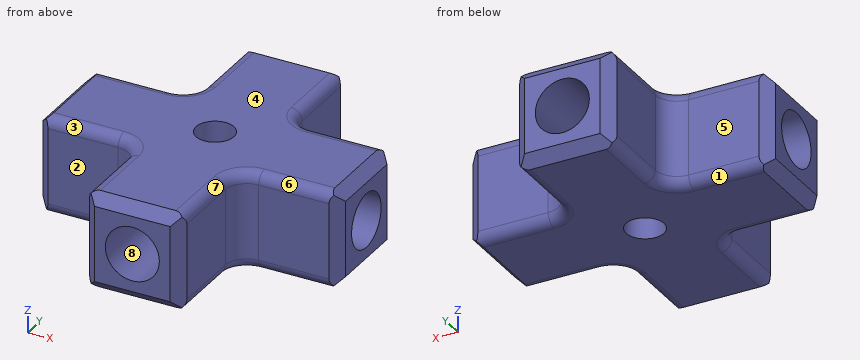
```python
from build123d import *

# Parameters (mm, degrees)
F0_W     = 9
F0_H     = 9.5
F0_W_2   = 9.5
F0_H_2   = 9
F0_R     = 1.75
F1_DEPTH = 9
F4_R     = 2.5
F6_DEPTH = 6.5
F3_R     = 2.5
F7_DEPTH = 6.5
F5_R     = 2.5
F8_DEPTH = 6.5
F2_R     = 2.5
F9_DEPTH = 6.5
F10_R    = 2
F11_SIZE = 1
F12_R    = 1


with BuildPart() as f1:
    # F0 (on Top) → F1 (new body)
    with BuildSketch(Plane.XY):
        with Locations((0, -9.25)):
            Rectangle(F0_W, F0_H)
        with Locations((9.25, 0)):
            Rectangle(F0_W_2, F0_H_2)
        with Locations((-9.25, 0)):
            Rectangle(F0_W_2, F0_H_2)
        with Locations((0, 9.25)):
            Rectangle(F0_W, F0_H)
        Rectangle(F0_W, F0_H_2)
        Circle(F0_R, mode=Mode.SUBTRACT)
    extrude(amount=F1_DEPTH)

    # F4 (on face) → F6 (cut)
    with BuildSketch(Plane(origin=(-14, 0, 0), x_dir=(0, -1, 0), z_dir=(-1, 0, 0))):
        with Locations((0, 4.4999998063)):
            Circle(F4_R)
    extrude(amount=-F6_DEPTH, mode=Mode.SUBTRACT)

    # F3 (on face) → F7 (cut)
    with BuildSketch(Plane.YZ.offset(14)):
        with Locations((0, 4.5)):
            Circle(F3_R)
    extrude(amount=-F7_DEPTH, mode=Mode.SUBTRACT)

    # F5 (on face) → F8 (cut)
    with BuildSketch(Plane.XZ.offset(14)):
        with Locations((0, 4.5042946003)):
            Circle(F5_R)
    extrude(amount=-F8_DEPTH, mode=Mode.SUBTRACT)

    # F2 (on face) → F9 (cut)
    with BuildSketch(Plane(origin=(0, 14, 0), x_dir=(-1, 0, 0), z_dir=(0, 1, 0))):
        with Locations((0, 4.5)):
            Circle(F2_R)
    extrude(amount=-F9_DEPTH, mode=Mode.SUBTRACT)

    # F10
    f10_edges = [f1.edges().sort_by_distance(p)[0] for p in [
        (-4.5, 4.5, 4.5),
        (-4.5, -4.5, 4.5),
        (4.5, -4.5, 4.5),
        (4.5, 4.5, 4.5),
    ]]
    fillet(f10_edges, radius=F10_R)

    # F11
    f11_edges = [f1.edges().sort_by_distance(p)[0] for p in [
        (14, 4.5, 4.5),
        (4.5, 14, 4.5),
        (-4.5, 14, 4.5),
        (-14, 4.5, 4.5),
        (-14, -4.5, 4.5),
        (-4.5, -14, 4.5),
        (4.5, -14, 4.5),
        (14, -4.5, 4.5),
        (14, 0, 0),
        (0, 14, 0),
        (-14, 0, 0),
        (0, -14, 0),
        (-14, 0, 9),
        (0, 14, 9),
        (0, -14, 9),
        (14, 0, 9),
    ]]
    chamfer(f11_edges, length=F11_SIZE)

    # F12
    f12_edges = [f1.edges().sort_by_distance(p)[0] for p in [
        (-9.75, -4.5, 9),
        (-9.75, 4.5, 9),
        (-4.5, -9.75, 9),
        (4.5, -9.75, 9),
        (9.75, -4.5, 9),
        (9.75, 4.5, 9),
        (4.5, 9.75, 9),
        (-4.5, 9.75, 9),
        (-9.75, 4.5, 0),
        (-9.75, -4.5, 0),
        (-4.5, -9.75, 0),
        (4.5, -9.75, 0),
        (9.75, -4.5, 0),
        (9.75, 4.5, 0),
        (4.5, 9.75, 0),
        (-4.5, 9.75, 0),
    ]]
    fillet(f12_edges, radius=F12_R)


solid = f1.part
```
Geometry: final body of the model. Coordinates: model frame, mm. Face numbers are marked on the shaded views. A direction names the side the tool comes from. Coordinates: 2 decimals unless noted, no trailing zeros. Order: outer loops, then holes, each group sorted by start corner. A loop starts at its lowest first (then second) coordinate and runs counter-clockwise, first axis right, second up. Notation, with made-up numbers: (37, 8) -> (58, 8) arc R25 cw to (58, 21) -> close; hole circle Ø10 at (7, 72.25). An arc over 180 degrees is marked (long way). Use CSV: the item, a comma, the result in double quotes.
1) Line query: line 1 (Z direction, x = -12.25, y = 0); line 2 (Y direction, x = -12, z = 4.5); line 3 (X direction, y = 10.5, z = 7.5). Output: solid intervals per line, ascending.
Findings:
line 1,"z = 0 to 2, 7 to 9"
line 2,"y = -4.5 to -2.5, 2.5 to 4.5"
line 3,"x = -4.5 to 4.5"
2) Section B-B on z = 7.5. Output: boundary loops of the cut face in (x, y), then the cut area to 3 significant figures.
Findings:
outline,"(-14, -3.5) -> (-13, -4.5) -> (-6.5, -4.5) arc R2 cw to (-4.5, -6.5) -> (-4.5, -13) -> (-3.5, -14) -> (3.5, -14) -> (4.5, -13) -> (4.5, -6.5) arc R2 cw to (6.5, -4.5) -> (13, -4.5) -> (14, -3.5) -> (14, 3.5) -> (13, 4.5) -> (6.5, 4.5) arc R2 cw to (4.5, 6.5) -> (4.5, 13) -> (3.5, 14) -> (-3.5, 14) -> (-4.5, 13) -> (-4.5, 6.5) arc R2 cw to (-6.5, 4.5) -> (-13, 4.5) -> (-14, 3.5) -> close; hole circle Ø3.5 at (0, 0)"
area,"413 mm^2"
3) Section A-A on x = 0. Output: boundary loops of the cut face in (y, z).
Findings:
outline,"(-14, 1) -> (-13, 0) -> (-1.75, 0) -> (-1.75, 9) -> (-13, 9) -> (-14, 8) -> (-14, 7) -> (-7.5, 7) -> (-7.5, 2) -> (-14, 2) -> close; (1.75, 0) -> (13, 0) -> (14, 1) -> (14, 2) -> (7.5, 2) -> (7.5, 7) -> (14, 7) -> (14, 8) -> (13, 9) -> (1.75, 9) -> close"
4) Mould query, pull axis X, two halves, no side actions, for the marked faces 6, 7 and 8. Classes: +X half, -X half, draft (parallel to the pull), parting line (faces both ways), or undercut.
Findings:
face 6,"draft"
face 7,"+X half"
face 8,"undercut"
5) Pin query (flat end, axial travel): pin 1 Ø5 at (x, z) = (-11, 3.5) entering from +Y; pin 2 Ø3 at (y, z) = (10.5, 3) entering from +X; pin 3 Ø3 at (y, z) = (0, 4.5) entering from -X. Return the tip coordinate at first contact, or that it passes through.
Findings:
pin 1,"stops at y = 4.5"
pin 2,"stops at x = 4.5"
pin 3,"stops at x = -7.5"
6) Access query for the marked faces 1, 2, 3, 4 and 5. Directions: +Z, -Z, +X, -X, +Y, -Y. A direction counts if a zero-diameter tool reaches every point of the face in a straight line with its end or side. Return the directions, or none.
Findings:
face 1,"-Z, -X, +Y"
face 2,"+Z, -Z, -X, -Y"
face 3,"+Z, -X, -Y"
face 4,"+Z, +X, -X, +Y, -Y"
face 5,"+Z, -Z, -X, +Y"
